from build123d import *

# Parameters (mm, degrees)
ESQUISSE1_R          = 2.1
BASE_EXTRUSION_DEPTH = 0.5


with BuildPart() as part:
    # Esquisse1 → Base-Extrusion (new, symmetric)
    with BuildSketch(Plane.XY):
        with BuildLine():
            Line((35.615327088, -25.672223926), (33.690495331, -5.355736059))
            ThreePointArc((33.690495331, -5.355736059), (32.627582421, 0.138570374), (30.529161577, 5.326423206))
            Line((30.529161577, 5.326423206), (20.291189648, 24.943575231))
            ThreePointArc((20.291189648, 24.943575231), (19.367522251, 26.19363098), (18.105897834, 27.101433088))
            Line((18.105897834, 27.101433088), (1.120998661, 35.694422442))
            ThreePointArc((1.120998661, 35.694422442), (-9.646140892, 36.898255889), (-18.57139047, 30.756559943))
            Line((-18.57139047, 30.756559943), (-21.986449586, 26.007166333))
            Line((-21.986449586, 26.007166333), (-33.307069298, 21.886797725))
            ThreePointArc((-33.307069298, 21.886797725), (-35.52580407, 20.184302655), (-36.366774139, 17.517086354))
            Line((-36.366774139, 17.517086354), (-36.366774139, 5.469934486))
            Line((-36.366774139, 5.469934486), (-39.661725259, 0.636440352))
            ThreePointArc((-39.661725259, 0.636440352), (-42.380416479, -9.851134542), (-37.566604459, -19.557200839))
            Line((-37.566604459, -19.557200839), (-23.682658123, -32.578809807))
            ThreePointArc((-23.682658123, -32.578809807), (-22.398102217, -33.453862354), (-20.907521199, -33.894281545))
            Line((-20.907521199, -33.894281545), (1.028164427, -36.805367071))
            ThreePointArc((1.028164427, -36.805367071), (6.620853648, -37.002887485), (12.147350486, -36.122535429))
            Line((12.147350486, -36.122535429), (31.896935448, -30.982637535))
            ThreePointArc((31.896935448, -30.982637535), (34.733377642, -29.011706008), (35.615327088, -25.672223926))
        make_face()
        with Locations((15.838548739, 22.619791811)):
            Circle(ESQUISSE1_R, mode=Mode.SUBTRACT)
        with Locations((-31.716624427, 17.517086354)):
            Circle(ESQUISSE1_R, mode=Mode.SUBTRACT)
        with Locations((-20.246771948, -28.915387001)):
            Circle(ESQUISSE1_R, mode=Mode.SUBTRACT)
        with Locations((30.63761742, -26.143823826)):
            Circle(ESQUISSE1_R, mode=Mode.SUBTRACT)
    extrude(amount=BASE_EXTRUSION_DEPTH, both=True)


solid = part.part
Could you check a few things on this model? Use its own coordinates, in mm. Give positions to 0.01 mm unless a question says otherwise; leave off trailing zeros. Order: outer loops, then holes, each group sorted by start corner. A loop starts at its lowest first (then second) coordinate and runs counter-clockwise, first axis right, second up. Notation, with made-up numbers: (57, -35.75) - (98, -35.75) arc R27 ccw to (98, -8.75) - close; hole circle Ø1 at (76.5, 65.5). An arc over 180 degrees is marked (long way). One line per item, written item: value. Start each with the question number.
1. Imagine slicing it at C-C on y = 1.5. List the corners of the cut face in (x, z) for me.
2. Imagine slicing it at B-B on x = 10.5. List the corners of the cut face in (y, z) for me.
3. Thinking about a two-plate mould opening in X: for faces 1 (the face through (19.38, 26.18, 0.01)), 2 (the face through (-42.396, -9.697, 0.007)), 3 (the face through (-33.815, 17.609, -0.007)), 4 (the face through (-22.345, -28.823, -0.007)), which applies, +X half, -X half, draft (parallel to the pull), parting line (faces both ways), or undercut?
4. Imagine slicing it at A-A on z = -0.3. List the corners of the cut face in (x, y) for me, plus the area to 3 significant figures.
5. For P1, Ø0.5, axis at y = 10, z = 0, coming from the -X side; P2, Ø4, axis at x = 30.64, y = -26.14, coming from the +Z side, each with a flat end and sliding along its axis, tell me the tip position at first contact or that it passes through.
6. If I drill on probe 1 along Y at (x, z) = (14, 0.05); probe 2 along X at (y, z) = (-26.5, -0.05); probe 3 along Y at (x, z) = (-20, -0.4), over which ranges is the centre line in solid material (lowest first)?
Values:
1. outline: (-39.07, -0.5) - (32.19, -0.5) - (32.19, 0.5) - (-39.07, 0.5) - close
2. outline: (-36.5, -0.5) - (30.95, -0.5) - (30.95, 0.5) - (-36.5, 0.5) - close
3. face 1: +X half
3. face 2: -X half
3. face 3: undercut
3. face 4: undercut
4. outline: (-39.66, 0.64) arc R15.5 ccw to (-37.57, -19.56) - (-23.68, -32.58) arc R5.02 ccw to (-20.91, -33.89) - (1.03, -36.81) arc R29 ccw to (12.15, -36.12) - (31.9, -30.98) arc R5 ccw to (35.62, -25.67) - (33.69, -5.36) arc R29 ccw to (30.53, 5.33) - (20.29, 24.94) arc R5.02 ccw to (18.11, 27.1) - (1.12, 35.69) arc R15.5 ccw to (-18.57, 30.76) - (-21.99, 26.01) - (-33.31, 21.89) arc R4.65 ccw to (-36.37, 17.52) - (-36.37, 5.47) - close; hole circle Ø4.2 at (-31.72, 17.52); hole circle Ø4.2 at (-20.25, -28.92); hole circle Ø4.2 at (15.84, 22.62); hole circle Ø4.2 at (30.64, -26.14)
4. area: 4,300 mm²
5. P1: x = -36.37
5. P2: through
6. probe 1: -35.64 to 21.61, 23.63 to 29.18
6. probe 2: -30.16 to 28.57, 32.71 to 35.62
6. probe 3: -34.01 to -31, -26.83 to 28.77
